Build history of the part. All positions in model axes, mm. A direction names the side the tool comes from. Give positions to 0.01 mm unless a question says otherwise; leave off trailing zeros. Loops run counter-clockwise (first coordinate to the right, second up) from the corner with the lowest first, then second, coordinate; pieces in that order, holes last. Notation, with made-up numbers: (32, 17) -> (37, 17) arc R22 cw to (37, 35) -> close; hole circle Ø6 at (71.25, -8.5). An arc over 180 degrees is marked (long way). Answer as a JSON object with one key per item and string values. Group by question number.
from build123d import *

# Parameters (mm, degrees)
SKETCH1_W             = 20
SKETCH1_H             = 20
BOSS_EXTRUDE1_DEPTH   = 10
SKETCH2_W             = 15.7
SKETCH2_H             = 15.7
BOSS_EXTRUDE2_DEPTH   = 3
CHAMFER1_SIZE         = 1
CHAMFER1_SIZE2        = 0.577350269
CHAMFER1_PART_2_SIZE  = 1
CHAMFER1_PART_2_SIZE2 = 0.577350269
CHAMFER1_PART_3_SIZE  = 1
CHAMFER1_PART_3_SIZE2 = 0.577350269
CHAMFER1_PART_4_SIZE  = 1
CHAMFER1_PART_4_SIZE2 = 0.577350269
CUT_EXTRUDE1_DEPTH    = 8
CHAMFER2_SIZE         = 1
CHAMFER2_SIZE2        = 2.747477419


with BuildPart() as part:
    # Sketch1 → Boss-Extrude1 (new body)
    with BuildSketch(Plane(origin=(0, 0, 0), x_dir=(1, 0, 0), z_dir=(0, 1, 0))):
        Rectangle(SKETCH1_W, SKETCH1_H)
    extrude(amount=BOSS_EXTRUDE1_DEPTH)

    # Sketch2 → Boss-Extrude2 (add)
    with BuildSketch(Plane(origin=(0, 10, 0), x_dir=(1, 0, 0), z_dir=(0, 1, 0))):
        Rectangle(SKETCH2_W, SKETCH2_H)
    extrude(amount=BOSS_EXTRUDE2_DEPTH)

    # Chamfer1
    chamfer1_edges = [part.edges().sort_by_distance(p)[0] for p in [
        (-7.85, 13, 0),
    ]]
    chamfer1_side = [part.faces().sort_by_distance(p)[0] for p in [
        (-7.85, 11.5, 0),
    ]]
    chamfer(chamfer1_edges, length=CHAMFER1_SIZE, length2=CHAMFER1_SIZE2, reference=chamfer1_side[0])

    # Chamfer1 part 2
    chamfer1_part_2_edges = [part.edges().sort_by_distance(p)[0] for p in [
        (0, 13, 7.85),
    ]]
    chamfer1_part_2_side = [part.faces().sort_by_distance(p)[0] for p in [
        (0, 11.5, 7.85),
    ]]
    chamfer(chamfer1_part_2_edges, length=CHAMFER1_PART_2_SIZE, length2=CHAMFER1_PART_2_SIZE2, reference=chamfer1_part_2_side[0])

    # Chamfer1 part 3
    chamfer1_part_3_edges = [part.edges().sort_by_distance(p)[0] for p in [
        (7.85, 13, 0),
    ]]
    chamfer1_part_3_side = [part.faces().sort_by_distance(p)[0] for p in [
        (7.85, 11.5, 0),
    ]]
    chamfer(chamfer1_part_3_edges, length=CHAMFER1_PART_3_SIZE, length2=CHAMFER1_PART_3_SIZE2, reference=chamfer1_part_3_side[0])

    # Chamfer1 part 4
    chamfer1_part_4_edges = [part.edges().sort_by_distance(p)[0] for p in [
        (0, 13, -7.85),
    ]]
    chamfer1_part_4_side = [part.faces().sort_by_distance(p)[0] for p in [
        (0, 11.5, -7.85),
    ]]
    chamfer(chamfer1_part_4_edges, length=CHAMFER1_PART_4_SIZE, length2=CHAMFER1_PART_4_SIZE2, reference=chamfer1_part_4_side[0])

    # Sketch3 → Cut-Extrude1 (cut)
    with BuildSketch(Plane.XZ):
        Polygon((-3.7, 6.408587988), (-7.4, 0), (-3.7, -6.408587988), (3.7, -6.408587988), (7.4, 0), (3.7, 6.408587988), align=None)
    extrude(amount=-CUT_EXTRUDE1_DEPTH, mode=Mode.SUBTRACT)

    # Chamfer2
    chamfer2_edges = [part.edges().sort_by_distance(p)[0] for p in [
        (0, 0, 6.408587988),
        (-5.55, 0, 3.204293994),
        (-5.55, 0, -3.204293994),
        (0, 0, -6.408587988),
        (5.55, 0, -3.204293994),
        (5.55, 0, 3.204293994),
    ]]
    chamfer2_side = [part.faces().sort_by_distance(p)[0] for p in [
        (0, 0, 9.717157288),
    ]]
    chamfer(chamfer2_edges, length=CHAMFER2_SIZE, length2=CHAMFER2_SIZE2, reference=chamfer2_side[0])


solid = part.part
(1) Saw through at B-B on x = 2.5. List the corners of the cut face in (y, z).
(2) 3-axis set-ups, long thin cutter, end or side, ignore diameter. For faces 1 (the flat face through (-10, 5, 0)), 2 (the flat face through (0, 11, 7.85)), 3 (the flat face through (-0.1, 1.4, -6.9)), 4 (the flat face through (7.85, 11, 0)): which of +Z, -Z, +X, -X, +Y, -Y reach the whole face in a straight line?
(3) Saw through at D-D on z = -8.5. List the corners of the cut face in (x, y).
(4) Probe line 1 along Z through (x, y) = (0.5, 4); line 2 along Y through (x, z) = (-5, 9); line 3 along Y through (x, z) = (5.25, -2). List the from-to ranges inside material, lowest first. Write a range as [from, to].
(5) Saw through at A-A on y = 6.25. List the corners of the cut face in (x, z).
(6) Pull direction X, two halves, no side cores. Call faces 5 (the flat face through (-9, 10, 0)), 6 (the flat face through (-5.524, 5.337, 3.249)), 7 (the flat face through (-7.85, 11, 0)): pulls with the +X half, pulls with the -X half, needs draft (parallel to the pull), parting line crosses it, or undercut.
(7) Pin check, flat tips, straight feed: pin 1 (1.6 mm diameter, centred on y = 11.5, z = 3, fed in from -X); pin 2 (6.5 mm diameter, centred on x = 1.5, z = -1, fed in from -Y); pin 3 (12 mm diameter, centred on x = 6.5, z = 2, fed in from -Y); pin 4 (1 mm diameter, centred on x = 3.5, y = 11, fed in from -Z). Stop position of each tip, or through.
(8) Saw through at C-C on z = -0.5. List the corners of the cut face in (x, y).
Calculated:
{
 "1": {"outline": "(0, -10) -> (10, -10) -> (10, -7.85) -> (12, -7.85) -> (13, -7.27) -> (13, 7.27) -> (12, 7.85) -> (10, 7.85) -> (10, 10) -> (0, 10) -> (0, 7.41) -> (2.75, 6.41) -> (8, 6.41) -> (8, -6.41) -> (2.75, -6.41) -> (0, -7.41) -> close"},
 "2": {"face 1": "+Z, -Z, -X, +Y, -Y", "face 2": "+Z, +X, -X, +Y", "face 3": "-Y", "face 4": "+Z, -Z, +X, +Y"},
 "3": {"outline": "(-10, 0) -> (10, 0) -> (10, 10) -> (-10, 10) -> close"},
 "4": {"line 1": "z = [-10, -6.41], [6.41, 10]", "line 2": "y = [0, 10]", "line 3": "y = [8, 13]"},
 "5": {"outline": "(-10, -10) -> (10, -10) -> (10, 10) -> (-10, 10) -> close; hole (-7.4, 0) -> (-3.7, -6.41) -> (3.7, -6.41) -> (7.4, 0) -> (3.7, 6.41) -> (-3.7, 6.41) -> close"},
 "6": {"face 5": "needs draft", "face 6": "undercut", "face 7": "pulls with the -X half"},
 "7": {"pin 1": "stops at x = -7.85", "pin 2": "stops at y = 8", "pin 3": "stops at y = 0", "pin 4": "stops at z = -7.85"},
 "8": {"outline": "(-10, 0) -> (-8.27, 0) -> (-7.11, 2.75) -> (-7.11, 8) -> (7.11, 8) -> (7.11, 2.75) -> (8.27, 0) -> (10, 0) -> (10, 10) -> (7.85, 10) -> (7.85, 12) -> (7.27, 13) -> (-7.27, 13) -> (-7.85, 12) -> (-7.85, 10) -> (-10, 10) -> close"}
}
